The drawing under review shows one solid part. Ordinate dimensions are in mm from its lowest x, y, z. A direction names the side the tool comes from. Give positions to 0.01 mm unless a question says otherwise; leave off trailing zeros. Order: outer loops, then holes, each group sorted by start corner. A loop starts at its lowest first (then second) coordinate and runs counter-clockwise, first axis right, second up. Notation, with made-up numbers: (18.25, 43.5) -> (63.25, 43.5) arc R8 cw to (63.25, 49.5) -> close; hole circle Ø4 at (72, 25.5). An arc over 180 degrees is marked (long way). Use a Markdown table: item, result. Add a question column.
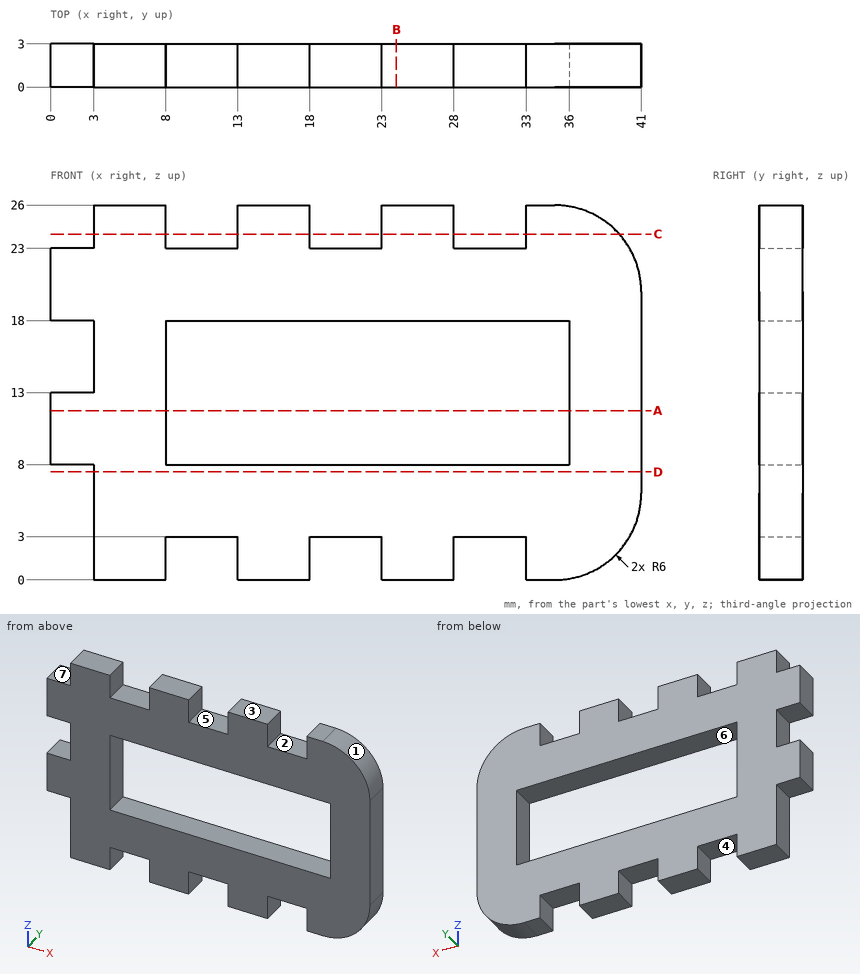
1) Insertion check: pin 1 (1.5 mm diameter, centred on x = 10, y = 2, fed in from +Z); pin 2 (0.9 mm diameter, centred on y = 1, z = 1.5, fed in from -X); pin 3 (1.5 mm diameter, centred on y = 1.5, z = 1, fed in from +X); pin 4 (6 mm diameter, centred on x = 28.5, z = 17.5, fed in from +Y). Each pin has a flat end and moves straight along its axis. Give the tip position at first contact, or say it passes through.
2) Machinability: for the marked faces 4, 5, 6 and 7, which of the approach directions +Z, -Z, +X, -X, +Y, -Y give a long, thin tool a straight path to every point of the face, cutting with its end or side? Answer none if there is none.
3) Add section A-A (z = 11.75). Give the boundary of the cut face in (x, y).
4) Add section C-C (z = 24). Give the boundary of the cut face in (x, y), then the cut area to 3 significant figures.
5) Add section B-B (x = 24). Give the boundary of the cut face in (y, z).
6) For L1, parallel to Z at x = 20.5, y = 1.65; L2, parallel to Z at x = 34, y = 1.35; L3, parallel to X at y = 1.45, z = 16, list the stretches that pass through material, from the lowest coordinate up. Write a range as [from, to].
7) The part is to be moulded in two halves that separate along X. For the marked faces 1, 2 and 3, say which applies: +X half, -X half, draft (parallel to the pull), parting line (faces both ways), or undercut.
8) Add section D-D (z = 7.5). Give the boundary of the cut face in (x, y).
Worked answers:
| question | item | result |
|---|---|---|
| 1 | pin 1 | z = 23 |
| 1 | pin 2 | x = 3 |
| 1 | pin 3 | x = 39.24 |
| 1 | pin 4 | y = 3 |
| 2 | face 4 | -Z, +Y, -Y |
| 2 | face 5 | +Z, +Y, -Y |
| 2 | face 6 | +Y, -Y |
| 2 | face 7 | +Z, -X, +Y, -Y |
| 3 | outline | (0, 0) -> (8, 0) -> (8, 3) -> (0, 3) -> close; (36, 0) -> (41, 0) -> (41, 3) -> (36, 3) -> close |
| 4 | outline | (3, 0) -> (8, 0) -> (8, 3) -> (3, 3) -> close; (13, 0) -> (18, 0) -> (18, 3) -> (13, 3) -> close; (23, 0) -> (28, 0) -> (28, 3) -> (23, 3) -> close; (33, 0) -> (39.47, 0) -> (39.47, 3) -> (33, 3) -> close |
| 4 | area | 64.4 mm^2 |
| 5 | outline | (0, 0) -> (3, 0) -> (3, 8) -> (0, 8) -> close; (0, 18) -> (3, 18) -> (3, 26) -> (0, 26) -> close |
| 6 | L1 | [3, 8], [18, 23] |
| 6 | L2 | [0, 8], [18, 26] |
| 6 | L3 | [3, 8], [36, 41] |
| 7 | face 1 | +X half |
| 7 | face 2 | undercut |
| 7 | face 3 | draft |
| 8 | outline | (3, 0) -> (41, 0) -> (41, 3) -> (3, 3) -> close |
